```python
from build123d import *

# Parameters (mm, degrees)
SKETCH1_R           = 1.6
BOSS_EXTRUDE1_DEPTH = 10
FILLET1_R           = 7.5
CHAMFER1_SIZE       = 1


with BuildPart() as part:
    # Sketch1 → Boss-Extrude1 (new body)
    with BuildSketch(Plane(origin=(0, 0, 0), x_dir=(1, 0, 0), z_dir=(0, 1, 0))):
        with BuildLine():
            Line((22.5, 57.5), (0, 57.5))
            Line((0, 57.5), (0, 102.5))
            Line((0, 102.5), (15, 102.5))
            Line((15, 102.5), (15, 72.5))
            Line((15, 72.5), (22.5, 72.5))
            ThreePointArc((22.5, 72.5), (43.713203436, 63.713203436), (52.5, 42.5))
            Line((52.5, 42.5), (52.5, -42.5))
            ThreePointArc((52.5, -42.5), (50.449747468, -47.449747468), (45.5, -49.5))
            Line((45.5, -49.5), (44.5, -49.5))
            ThreePointArc((44.5, -49.5), (39.550252532, -47.449747468), (37.5, -42.5))
            Line((37.5, -42.5), (37.5, 42.5))
            ThreePointArc((37.5, 42.5), (33.106601718, 53.106601718), (22.5, 57.5))
        make_face()
        with Locations(Location((9.4, 97.9, 0), (0, 0, 270))):
            Circle(SKETCH1_R, mode=Mode.SUBTRACT)
        with Locations(Location((9.4, 76.7, 0), (0, 0, 270))):
            Circle(SKETCH1_R, mode=Mode.SUBTRACT)
    extrude(amount=BOSS_EXTRUDE1_DEPTH)

    # Fillet1
    fillet1_edges = [part.edges().sort_by_distance(p)[0] for p in [
        (15, 5, -72.5),
    ]]
    fillet(fillet1_edges, radius=FILLET1_R - 0.0001)  # a hair under: the kernel refuses the full size

    # Chamfer1
    chamfer1_edges = [part.edges().sort_by_distance(p)[0] for p in [
        (7.5, 0, -102.5),
        (33.106601718, 10, -53.106601718),
        (43.713203436, 0, -63.713203436),
        (52.5, 0, 0),
        (50.449747468, 0, 47.449747468),
        (45, 0, 49.5),
        (39.550252532, 0, 47.449747468),
        (37.5, 0, 0),
        (33.106601718, 0, -53.106601718),
        (11.25, 0, -57.5),
        (37.5, 10, 0),
        (15, 5, -102.5),
        (39.550252532, 10, 47.449747468),
        (45, 10, 49.5),
        (50.449747468, 10, 47.449747468),
        (52.5, 10, 0),
        (43.713203436, 10, -63.713203436),
        (15, 0, -91.24995),
        (15, 10, -91.24995),
        (17.196669852, 0, -74.696669852),
        (17.196669852, 10, -74.696669852),
        (7.5, 10, -102.5),
        (11.25, 10, -57.5),
    ]]
    chamfer(chamfer1_edges, length=CHAMFER1_SIZE)

    # Mirror1: part across plane


with BuildPart() as part_1:
    add(part.part)
    add(part.part.mirror(Plane(origin=(0, 10, -57.5), x_dir=(0, 0, 1), z_dir=(1, 0, 0))))


solid = part_1.part
```
The listing builds one solid part. Answer for the finished solid, in the listing's coordinates (mm). A direction names the side the tool comes from. Give positions to 0.01 mm unless a question says otherwise; leave off trailing zeros. Loops run counter-clockwise (first coordinate to the right, second up) from the corner with the lowest first, then second, coordinate; pieces in that order, holes last. Notation, with made-up numbers: (0, 86) - (34, 86) arc R23 ccw to (34, 108) - close; hole circle Ø8 at (41, 57). An arc over 180 degrees is marked (long way). Answer as CSV lines item,"result". Start each with the question number.
Item 1: For faces 5 (the face through (-15, 5, -91)), 6 (the face through (33.34, 0.84, -53.1)), 7 (the face through (15, 5, -91)), 8 (the face through (33.22, 4.94, -52.99)), determine the directions among +Z, -Z, +X, -X, +Y, -Y from which every point of the face is accessible in a straight line to the end or side of a thin tool.
Item 2: Find the intervals of material crossed by line 1 (Z direction, x = -9.4, y = 7.25); line 2 (X direction, y = 6.5, z = -97.9); line 3 (X direction, y = 3.75, z = -76.7), in increasing order. Write a range as from..to.
Item 3: The mould has two halves that part along X. Classify faces 1 (the face through (-42.9, 9.83, -63.35)), 2 (the face through (0, 5, -102.5)), 3 (the face through (8.79, 4.93, -75.22)), 4 (the face through (-39.6, 4.9, 47.5)): +X half, -X half, draft (parallel to the pull), parting line (faces both ways), or undercut.
Item 4: A cutting plane is placed at D-D on x = -9.4. Determine the outline of the cut face in (y, z), then the cut area to 3 significant figures.
Item 5: A cutting plane is placed at C-C on z = -97.9. Determine the outline of the cut face in (x, y), then the cut area to 3 significant figures.
Item 6: A cutting plane is placed at A-A on z = -17. Determine the outline of the cut face in (x, y), then the cut area to 3 significant figures.
Item 7: Each of these flat-tipped pins is pushed along its axis until it touches: pin 1 (5 mm diameter, centred on x = -25, y = 1.5, fed in from +Z); pin 2 (3 mm diameter, centred on x = 9.4, z = -76.7, fed in from +Y); pin 3 (1 mm diameter, centred on x = 2, y = 7, fed in from +Z). Where does it stop, or does it pass through?
Item 8: A cutting plane is placed at B-B on y = 4.75. Count the separate pieces of the cut face and the enclosed holes in it, then the cut area to 3 significant figures.
Found:
1,face 5,"-Z, -X, +Y, -Y"
1,face 6,"+Z, -Y"
1,face 7,"-Z, +X, +Y, -Y"
1,face 8,"+Z, +Y, -Y"
2,line 1,"z = -102.5..-99.5, -96.3..-78.3, -75.1..-57.5"
2,line 2,"x = -15..-11, -7.8..7.8, 11..15"
2,line 3,"x = -15.76..-11, -7.8..7.8, 11..15.76"
3,face 1,"-X half"
3,face 2,"draft"
3,face 3,"undercut"
3,face 4,"undercut"
4,outline,"(0, -101.5) - (1, -102.5) - (9, -102.5) - (10, -101.5) - (10, -99.5) - (0, -99.5) - close; (0, -96.3) - (10, -96.3) - (10, -78.3) - (0, -78.3) - close; (0, -75.1) - (10, -75.1) - (10, -58.5) - (9, -57.5) - (1, -57.5) - (0, -58.5) - close"
4,area,"384 mm^2"
5,outline,"(-15, 1) - (-14, 0) - (-11, 0) - (-11, 10) - (-14, 10) - (-15, 9) - close; (-7.8, 0) - (7.8, 0) - (7.8, 10) - (-7.8, 10) - close; (11, 0) - (14, 0) - (15, 1) - (15, 9) - (14, 10) - (11, 10) - close"
5,area,"234 mm^2"
6,outline,"(-52.5, 1) - (-51.5, 0) - (-38.5, 0) - (-37.5, 1) - (-37.5, 9) - (-38.5, 10) - (-51.5, 10) - (-52.5, 9) - close; (37.5, 1) - (38.5, 0) - (51.5, 0) - (52.5, 1) - (52.5, 9) - (51.5, 10) - (38.5, 10) - (37.5, 9) - close"
6,area,"296 mm^2"
7,pin 1,"stops at z = -56.64"
7,pin 2,"passes through"
7,pin 3,"stops at z = -57.5"
8,separate pieces,"1"
8,enclosed holes,"4"
8,area,"5,340 mm^2"
